```python
from build123d import *

# Parameters (mm, degrees)
F0_R     = 85
F2_R     = 0.5
F4_R     = 105.9677495378
F5_DEPTH = 1


# Not quite as in the source:
# - a fillet or chamfer that OpenCascade refuses, or shapes differently, is made with other operations: its cross-section is extruded or revolved along the edge and cut away or added


with BuildPart() as f3:
    # F0 (on Top) → F3 section 0
    with BuildSketch(Plane.XY):
        Circle(F0_R)
    # F2 (on offset) → F3 section 1
    with BuildSketch(Plane.XY.offset(1300)):
        Circle(F2_R)
    loft()

    # F4 (on Top) → F5 (join)
    with BuildSketch(Plane.XY):
        Circle(F4_R)
    extrude(amount=F5_DEPTH)

    # F6: fillet of radius 50 on 1 edges, made by hand


with BuildPart() as f6_tool2:
    # F6_s3 → F6_t4 (revolve)
    with BuildSketch(Plane.XZ):
        with BuildLine():
            ThreePointArc((105.9675390616, 0.9996598533), (89.4115983215, 17.7775955554), (82.3816590809, 40.2760011541))
            Line((82.3816590809, 40.2760011541), (77.3920405677, 39.9516759507))
            ThreePointArc((77.3920405677, 39.9516759507), (78.6689106061, 20.3136883463), (79.9453814868, 0.6756747966))
            Line((79.9453814868, 0.6756747966), (84.935, -4.0001479723))
            ThreePointArc((84.935, -4.0001479723), (95.4512695308, -4.0001479723), (103.3365085465, -3.2522994801))
            Line((103.3365085465, -3.2522994801), (105.9675390616, 0.9996598533))
        make_face()
    revolve(axis=Axis((0, 0, 1), (0, 0, 1)))

    split(bisect_by=Plane.XY, keep=Keep.TOP)


with BuildPart() as f3_1:
    add(f3.part)

    # F6_t1: union F6_tool2
    add(f6_tool2.part)


solid = f3_1.part
```
CAD build for the part. Positions are in the model's coordinates, mm. Coordinates: 2 decimals unless noted, no trailing zeros. Order: outer loops, then holes, each group sorted by start corner. A loop starts at its lowest first (then second) coordinate and runs counter-clockwise, first axis right, second up. Notation, with made-up numbers: (3.25, -39) - (54.25, -39) arc R9 ccw to (54.25, -34) - close; hole circle Ø8 at (-3, -20). An arc over 180 degrees is marked (long way). Use a Markdown table: item, result. Add a question column.
(1) Saw through at A-A (z = 1118). Give the cut face in (x, y).
(2) Saw through at B-B (z = 494.5). Give the cut face in (x, y) (1 decimal), then the cut area to 3 significant figures.
(3) Drill centre lines: line 1 along Z through (x, y) = (67, 76); line 2 along X through (y, z) = (-4, 609); line 3 along Y through (x, z) = (-56, 166). Where is each one in solid material? Low to high. Write a range as [from, to].
(4) Flat gauge pins, fed straight in: pin 1 (12 mm diameter, centred on y = -11, z = 388.5, fed in from +X); pin 2 (4 mm diameter, centred on x = 61, z = 205, fed in from +Y); pin 3 (1 mm diameter, centred on y = 10, z = 1035.5, fed in from +X). Where does each tip first touch, or does it go through?
Solved:
| question | item | result |
|---|---|---|
| 1 | outline | circle Ø24.66 at (0, 0) |
| 2 | outline | circle Ø105.7 at (0, 0) |
| 2 | area | 8,780 mm² |
| 3 | line 1 | z = [0, 4.26] |
| 3 | line 2 | x = [-45.24, 45.24] |
| 3 | line 3 | y = [-48.69, 48.69] |
| 4 | pin 1 | stops at x = 59.66 |
| 4 | pin 2 | stops at y = 40.71 |
| 4 | pin 3 | stops at x = 14.93 |
